The model under review builds one solid part; all positions refer to its coordinate system, in mm. A direction names the side the tool comes from. Coordinates: 2 decimals unless noted, no trailing zeros. Order: outer loops, then holes, each group sorted by start corner. A loop starts at its lowest first (then second) coordinate and runs counter-clockwise, first axis right, second up. Notation, with made-up numbers: M 8,61 L 59,61 A23 cw 59,74 Z; hole C 10.25,47.5 d1. An arc over 180 degrees is marked long. Write each question's results on one line, items separated by ' | '.
from build123d import *

# Parameters (mm, degrees)
SKETCH1_R          = 1.5
BASE_EXTRUDE_DEPTH = 6
CUT_EXTRUDE1_DEPTH = 1.799999969
CUT_EXTRUDE1_TAPER = 2


with BuildPart() as part:
    # Sketch1 → Base-Extrude (new body)
    with BuildSketch(Plane.XY):
        Circle(SKETCH1_R)
    extrude(amount=BASE_EXTRUDE_DEPTH)

    # Sketch6 → Boss-Revolve2 (revolve)
    with BuildSketch(Plane(origin=(0, 0, 0), x_dir=(1, 0, 0), z_dir=(0, 1, 0))):
        with BuildLine():
            Line((0, -6), (2.7999999, -6))
            Line((2.7999999, -6), (2.7999999, -7.54246308))
            ThreePointArc((2.7999999, -7.54246308), (1.46418655, -8.180811406), (0, -8.4))
            Line((0, -8.4), (0, -6))
        make_face()
    revolve(axis=Axis((0, 0, -0.393620135), (0, 0, 1)))

    # Sketch7 → Cut-Extrude1 (cut)
    with BuildSketch(Plane(origin=(0, 0, 8.7000001), x_dir=(-1, 0, 0), z_dir=(0, 0, -1))):
        with BuildLine():
            ThreePointArc((0.205000004, 1.48592565), (0, 1.500000013), (-0.205000004, 1.48592565))
            Line((-0.205000004, 1.48592565), (-0.205000004, 0.708178558))
            ThreePointArc((-0.205000004, 0.708178558), (-0.35072876, 0.355344481), (-0.702967546, 0.208182689))
            Line((-0.702967546, 0.208182689), (-1.48592565, 0.205000004))
            ThreePointArc((-1.48592565, 0.205000004), (-1.500000013, 0), (-1.48592565, -0.205000004))
            Line((-1.48592565, -0.205000004), (-0.702967546, -0.208182689))
            ThreePointArc((-0.702967546, -0.208182689), (-0.35072876, -0.355344481), (-0.205000004, -0.708178558))
            Line((-0.205000004, -0.708178558), (-0.205000004, -1.48592565))
            ThreePointArc((-0.205000004, -1.48592565), (0, -1.500000013), (0.205000004, -1.48592565))
            Line((0.205000004, -1.48592565), (0.205000004, -0.708178558))
            ThreePointArc((0.205000004, -0.708178558), (0.35072876, -0.355344481), (0.702967546, -0.208182689))
            Line((0.702967546, -0.208182689), (1.48592565, -0.205000004))
            ThreePointArc((1.48592565, -0.205000004), (1.500000013, 0), (1.48592565, 0.205000004))
            Line((1.48592565, 0.205000004), (0.702967546, 0.208182689))
            ThreePointArc((0.702967546, 0.208182689), (0.35072876, 0.355344481), (0.205000004, 0.708178558))
            Line((0.205000004, 0.708178558), (0.205000004, 1.48592565))
        make_face()
    extrude(amount=CUT_EXTRUDE1_DEPTH, taper=CUT_EXTRUDE1_TAPER, mode=Mode.SUBTRACT)


solid = part.part
1) Take a section at B-B on y = -1.7. State the section outline as (x, z) points, plus the area to 3 significant figures.
Solutions:
outline: M -2.22,6 L 2.22,6 L 2.22,7.54 A4.7 ccw -2.22,7.54 Z | area: 8.54 mm2
2) To check wall thickness, follow line 1 along X through (y, z) = (-0.05, 5.75); line 2 along Y through (x, z) = (1.25, 7.75); line 3 along Z through (x, y) = (0, -1.6). State the ranges of each line that lie inside material, in increasing order.
Solutions:
line 1: -1.5 to 1.5 | line 2: -2.12 to -0.17, 0.17 to 2.12 | line 3: 6 to 8.14
3) Take a section at C-C on x = 1.8. State the section outline as (y, z) points, plus the area to 3 significant figures.
Solutions:
outline: M -2.14,6 L 2.14,6 L 2.14,7.54 A4.66 ccw -2.14,7.54 Z | area: 8.13 mm2
4) The part is to be moulded in two halves that separate along Y. For faces 3 (the flat face through (0, 0, 0)), 4 (the cylindrical face through (-1.5, 0.07, 2.96)), 5 (the flat face through (0, 0, 6.9)), say which applies: pulls with the +Y half, pulls with the -Y half, needs draft (parallel to the pull), parting line crosses it, or undercut.
Solutions:
face 3: needs draft | face 4: parting line crosses it | face 5: undercut
5) Take a section at A-A on z = 5.75. State the section outline as (x, y) points.
Solutions:
outline: C 0,0 d3
6) For faces 1 (the cylindrical face through (-0.607, -2.733, 6.782)), 2 (the flat face through (-1.2, -1.2, 6)), list the 3-axis set-ups (+Z, -Z, +X, -X, +Y, -Y) from which the entire face can be reached by the end or side of a thin tool; tool diameter is ignored.
Solutions:
face 1: +Z, -Z | face 2: -Z
7) For pin 1 (2 mm diameter, centred on y = 1.5, z = 7, fed in from -X) (3 decimals); pin 2 (1.5 mm diameter, centred on x = 1, z = 7.5, fed in from +Y), all flat-tipped, find the tip position at first contact; note any pin that passes through.
Solutions:
pin 1: x = -2.755 | pin 2: y = 2.79
